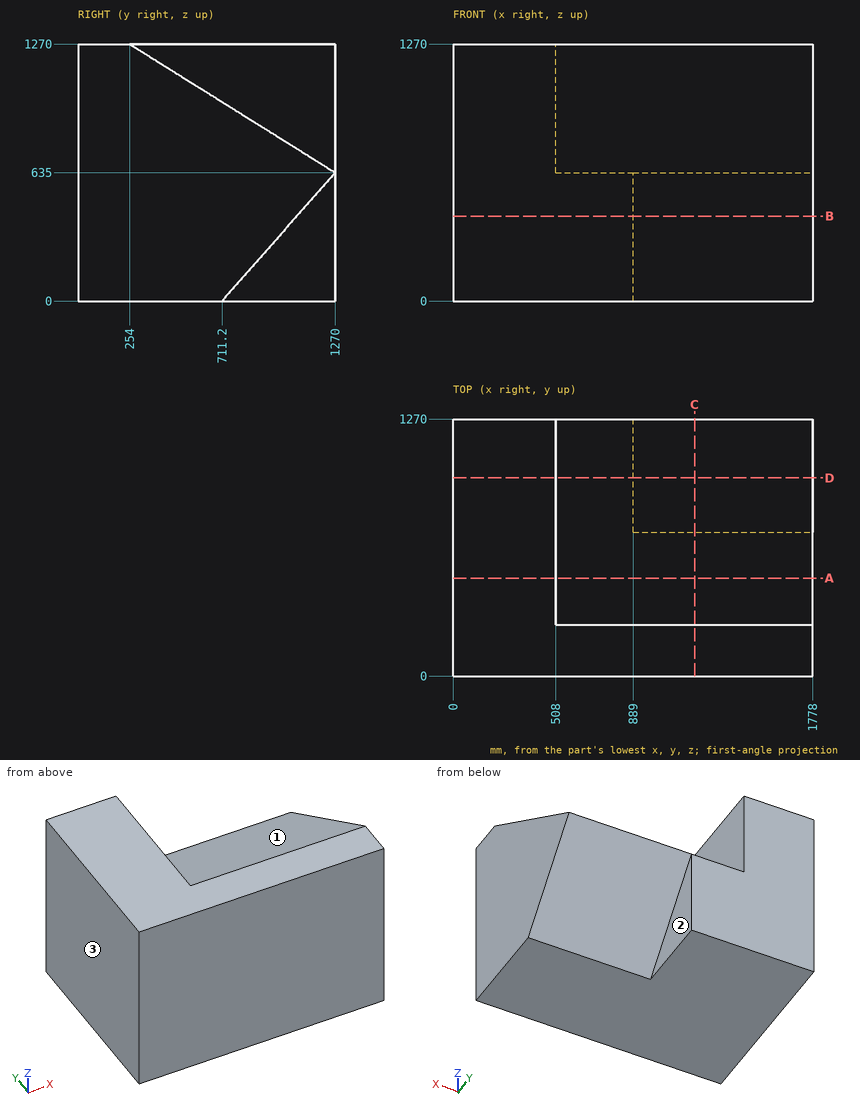
Print and shaded views of the part. All mm, measured from the part's lowest x, y and z. A direction names the side the tool comes from. Give positions to 0.01 mm unless a question says otherwise; leave off trailing zeros. Order: outer loops, then holes, each group sorted by start corner. A loop starts at its lowest first (then second) coordinate and runs counter-clockwise, first axis right, second up. Notation, with made-up numbers: (64, 89.5) - (110, 89.5) arc R20 cw to (110, 116.5) - close; hole circle Ø3 at (65, 81). An arc over 180 degrees is marked (long way). One line per item, written item: value.
Item 1: Slice it at B-B (z = 420). List the corners of the cut face in (x, y).
Response values:
outline: (0, 0) - (1778, 0) - (1778, 1080.8) - (889, 1080.8) - (889, 1270) - (0, 1270) - close
Item 2: Pin check, flat tips, straight feed: pin 1 Ø3 at (y, z) = (629, 433) entering from -X; pin 2 Ø4 at (x, y) = (1055, 746) entering from -Z; pin 3 Ø6 at (x, y) = (1038.5, 700) entering from +Z (3 decimals); pin 4 Ø8 at (x, y) = (1163.5, 1076) entering from -Z. Stop position of each tip, or through.
Response values:
pin 1: x = 0
pin 2: z = 37.27
pin 3: z = 993.125
pin 4: z = 410
Item 3: Slice it at C-C (x = 1194). List the corners of the cut face in (y, z), then the cut area to 3 significant figures.
Response values:
outline: (0, 0) - (711.2, 0) - (1270, 635) - (254, 1270) - (0, 1270) - close
area: 1,110,000 mm2
Item 4: Slice it at A-A (y = 484). List the corners of the cut face in (x, z), then the cut area to 3 significant figures.
Response values:
outline: (0, 0) - (1778, 0) - (1778, 1126.25) - (508, 1126.25) - (508, 1270) - (0, 1270) - close
area: 2,080,000 mm2
Item 5: Slice it at D-D (y = 979.5). List the corners of the cut face in (x, z).
Response values:
outline: (0, 0) - (889, 0) - (889, 304.89) - (1778, 304.89) - (1778, 816.56) - (508, 816.56) - (508, 1270) - (0, 1270) - close
Item 6: Tool access for the marked faces 1, 2 and 3: list every direction of +Z, -Z, +X, -X, +Y, -Y with a clear straight run to the whole face (end or side of a thin tool).
Response values:
face 1: +Z, +X, +Y
face 2: -Z, +X, +Y
face 3: +Z, -Z, -X, +Y, -Y
Item 7: Wall check: line 1 (X direction, y = 1082.5, z = 265.5); line 2 (Z direction, x = 1019, y = 541) (3 decimals); line 3 (Z direction, x = 1011.5, y = 675) (3 decimals). Give the ranges that are in metal, low to high.
Response values:
line 1: 0 to 889
line 2: 0 to 1090.625
line 3: 0 to 1006.875
